Geometry check sheet. Reference: the model listing, model coordinates, mm. Coordinates: 2 decimals unless noted, no trailing zeros. Loops run counter-clockwise (first coordinate to the right, second up) from the corner with the lowest first, then second, coordinate; pieces in that order, holes last.
from build123d import *

# Parameters (mm, degrees)
SKETCH1_W           = 93
SKETCH1_H           = 61
SKETCH1_R           = 2
SKETCH1_R_2         = 1.5
SKETCH1_W_2         = 12
SKETCH1_H_2         = 20.75
SKETCH1_W_3         = 40
SKETCH1_W_4         = 15
BOSS_EXTRUDE1_DEPTH = 1.5


with BuildPart() as part:
    # Sketch1 → Boss-Extrude1 (new, symmetric)
    with BuildSketch(Plane(origin=(0, 0, 0), x_dir=(1, 0, 0), z_dir=(0, 1, 0))):
        Rectangle(SKETCH1_W, SKETCH1_H)
        with Locations(Location((-34, 0, 0), (0, 0, 270))):
            Circle(SKETCH1_R, mode=Mode.SUBTRACT)
        with Locations(Location((-14, 0, 0), (0, 0, 270))):
            Circle(SKETCH1_R, mode=Mode.SUBTRACT)
        with Locations(Location((16, 0, 0), (0, 0, 270))):
            Circle(SKETCH1_R, mode=Mode.SUBTRACT)
        with Locations(Location((43.25, -27.25, 0), (0, 0, 270))):
            Circle(SKETCH1_R_2, mode=Mode.SUBTRACT)
        with Locations(Location((-43.25, -27.25, 0), (0, 0, 270))):
            Circle(SKETCH1_R_2, mode=Mode.SUBTRACT)
        with Locations(Location((43.25, 27.25, 0), (0, 0, 90))):
            Circle(SKETCH1_R_2, mode=Mode.SUBTRACT)
        with Locations(Location((-43.25, 27.25, 0), (0, 0, 90))):
            Circle(SKETCH1_R_2, mode=Mode.SUBTRACT)
        with Locations((-34, -13.625)):
            Rectangle(SKETCH1_W_2, SKETCH1_H_2, mode=Mode.SUBTRACT)
        with Locations((-34, 13.625)):
            Rectangle(SKETCH1_W_2, SKETCH1_H_2, mode=Mode.SUBTRACT)
        with Locations((20, -13.625)):
            Rectangle(SKETCH1_W_3, SKETCH1_H_2, mode=Mode.SUBTRACT)
        with Locations((-14, 13.625)):
            Rectangle(SKETCH1_W_4, SKETCH1_H_2, mode=Mode.SUBTRACT)
        with Locations((20, 13.625)):
            Rectangle(SKETCH1_W_3, SKETCH1_H_2, mode=Mode.SUBTRACT)
        with Locations((-14, -13.625)):
            Rectangle(SKETCH1_W_4, SKETCH1_H_2, mode=Mode.SUBTRACT)
    extrude(amount=BOSS_EXTRUDE1_DEPTH, both=True)


solid = part.part
1) Mould release check, pull along Z, two halves, no side actions. Record for faces 1 (the flat face through (-1, -1.5, 0)), 2 (the flat face through (-1, 0, -30.5)), 3 (the flat face through (-34, 0, -3.25)), 4 (the flat face through (-40, 0, 14)): +Z half, -Z half, draft (parallel to the pull), parting line (faces both ways), or undercut.
Data:
face 1: draft
face 2: -Z half
face 3: undercut
face 4: undercut
2) Section check B-B on z = 6. Record the cut outline in (x, y), and give its area (3 significant figures).
Data:
outline: (-46.5, -1.5) - (-40, -1.5) - (-40, 1.5) - (-46.5, 1.5) - close; (-28, -1.5) - (-21.5, -1.5) - (-21.5, 1.5) - (-28, 1.5) - close; (-6.5, -1.5) - (0, -1.5) - (0, 1.5) - (-6.5, 1.5) - close; (40, -1.5) - (46.5, -1.5) - (46.5, 1.5) - (40, 1.5) - close
area: 78.0 mm2
3) Section check C-C on x = -34. Record the cut outline in (y, z), and give its area (3 significant figures).
Data:
outline: (-1.5, -30.5) - (1.5, -30.5) - (1.5, -24) - (-1.5, -24) - close; (-1.5, -3.25) - (1.5, -3.25) - (1.5, -2) - (-1.5, -2) - close; (-1.5, 2) - (1.5, 2) - (1.5, 3.25) - (-1.5, 3.25) - close; (-1.5, 24) - (1.5, 24) - (1.5, 30.5) - (-1.5, 30.5) - close
area: 46.5 mm2
4) Section check D-D on z = 27.25. Record the cut outline in (x, y).
Data:
outline: (-46.5, -1.5) - (-44.75, -1.5) - (-44.75, 1.5) - (-46.5, 1.5) - close; (-41.75, -1.5) - (41.75, -1.5) - (41.75, 1.5) - (-41.75, 1.5) - close; (44.75, -1.5) - (46.5, -1.5) - (46.5, 1.5) - (44.75, 1.5) - close
5) Depth check by flat-ended pin: pin 1 (3.5 mm diameter, centred on x = 16, z = 0, fed in from +Y); pin 2 (5 mm diameter, centred on x = -14, z = 0, fed in from +Y). Enter the tip coordinate at first touch or a pass-through.
Data:
pin 1: passes through
pin 2: stops at y = 1.5
6) Section check A-A on x = 9.5. Record the cut outline in (y, z).
Data:
outline: (-1.5, -30.5) - (1.5, -30.5) - (1.5, -24) - (-1.5, -24) - close; (-1.5, -3.25) - (1.5, -3.25) - (1.5, 3.25) - (-1.5, 3.25) - close; (-1.5, 24) - (1.5, 24) - (1.5, 30.5) - (-1.5, 30.5) - close
7) Material ranges on probe 1 along X at (y, z) = (0.65, -16); probe 2 along X at (y, z) = (0, -27.25); probe 3 along X at (y, z) = (0.1, 0), recorded low to high.
Data:
probe 1: x = -46.5 to -40, -28 to -21.5, -6.5 to 0, 40 to 46.5
probe 2: x = -46.5 to -44.75, -41.75 to 41.75, 44.75 to 46.5
probe 3: x = -46.5 to -36, -32 to -16, -12 to 14, 18 to 46.5
